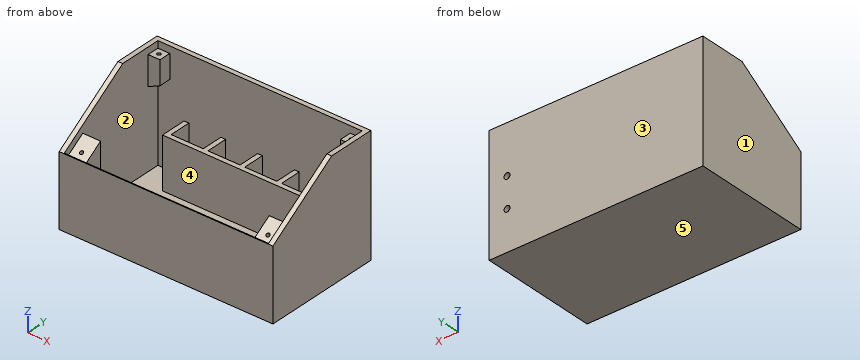
from build123d import *

# Parameters (mm, degrees)
ESBO_O1_W                = 180
ESBO_O1_H                = 100
ESBO_O1_W_2              = 172
ESBO_O1_H_2              = 92
RESSALTO_EXTRUS_O1_DEPTH = 100
ESBO_O2_W                = 180
ESBO_O2_H                = 100
RESSALTO_EXTRUS_O2_DEPTH = 4
RESSALTO_EXTRUS_O3_DEPTH = 43
CORTE_EXTRUS_O1_DEPTH    = 263
CHANFRO1_SIZE            = 6
CHANFRO1_SIZE2           = 4.326661531
ESBO_O5_W                = 10
ESBO_O5_H                = 20
RESSALTO_EXTRUS_O4_DEPTH = 10
ESBO_O6_R                = 1.5
CORTE_EXTRUS_O2_DEPTH    = 32
ESBO_O7_R                = 2.5
CORTE_EXTRUS_O3_DEPTH    = 32
CHANFRO3_SIZE            = 4.663076582
CHANFRO3_SIZE_2          = 10
CHANFRO4_SIZE            = 10
CHANFRO4_SIZE_2          = 4.663076582
RESSALTO_EXTRUS_O5_DEPTH = 15
RESSALTO_EXTRUS_O6_DEPTH = 15
CHANFRO5_SIZE2           = 15
CHANFRO5_SIZE            = 6.994614872
CHANFRO6_SIZE2           = 15
CHANFRO6_SIZE            = 6.994614872
ESBO_O10_R               = 1.5
CORTE_EXTRUS_O4_DEPTH    = 5
ESBO_O11_W               = 11
ESBO_O11_H               = 26
ESBO_O11_R               = 2
RESSALTO_EXTRUS_O7_DEPTH = 5


# Some blends are built 0.0001 mm under size
with BuildPart() as part:
    # Esboço1 → Ressalto-extrusão1 (new body)
    with BuildSketch(Plane.XY):
        with Locations((90, 50)):
            Rectangle(ESBO_O1_W, ESBO_O1_H)
        with Locations((90, 50)):
            Rectangle(ESBO_O1_W_2, ESBO_O1_H_2, mode=Mode.SUBTRACT)
    extrude(amount=RESSALTO_EXTRUS_O1_DEPTH)

    # Esboço2 → Ressalto-extrusão2 (add)
    with BuildSketch(Plane(origin=(0, 0, 0), x_dir=(-1, 0, 0), z_dir=(0, 0, -1))):
        with Locations((-90, 50)):
            Rectangle(ESBO_O2_W, ESBO_O2_H)
    extrude(amount=-RESSALTO_EXTRUS_O2_DEPTH)

    # Esboço3 → Ressalto-extrusão3 (add)
    with BuildSketch(Plane.XY.offset(4)):
        Polygon((30, 96), (30, 78), (57, 78), (57, 96), (61, 96), (61, 78), (88, 78), (88, 96), (92, 96), (92, 78), (119, 78), (119, 96), (123, 96), (123, 78), (150, 78), (150, 96), (154, 96), (154, 74), (26, 74), (26, 96), align=None)
    extrude(amount=RESSALTO_EXTRUS_O3_DEPTH)

    # Esboço4 → Corte-extrusão1 (cut)
    with BuildSketch(Plane.ZY):
        Polygon((60, 0), (100, 60), (100, 0), align=None)
    extrude(amount=-CORTE_EXTRUS_O1_DEPTH, mode=Mode.SUBTRACT)

    # Chanfro1
    chanfro1_edges = [part.edges().sort_by_distance(p)[0] for p in [
        (90, 4, 62.666666667),
    ]]
    chanfro1_side = [part.faces().sort_by_distance(p)[0] for p in [
        (90, 4, 33.333333333),
    ]]
    chamfer(chanfro1_edges, length=CHANFRO1_SIZE, length2=CHANFRO1_SIZE2, reference=chanfro1_side[0])

    # Esboço5 → Ressalto-extrusão4 (add)
    with BuildSketch(Plane.XZ.offset(-96)):
        with Locations((9, 84.2)):
            Rectangle(ESBO_O5_W, ESBO_O5_H)
        with Locations((171, 84.2)):
            Rectangle(ESBO_O5_W, ESBO_O5_H)
    extrude(amount=RESSALTO_EXTRUS_O4_DEPTH)

    # Esboço6 → Corte-extrusão2 (cut)
    with BuildSketch(Plane.XY.offset(94.2)):
        with Locations((171, 91)):
            Circle(ESBO_O6_R)
        with Locations((9, 91)):
            Circle(ESBO_O6_R)
    extrude(amount=-CORTE_EXTRUS_O2_DEPTH, mode=Mode.SUBTRACT)

    # Esboço7 → Corte-extrusão3 (cut)
    with BuildSketch(Plane.XZ.offset(-96)):
        with Locations(Location((165, 58.88, 0), (0, 0, 270))):
            Circle(ESBO_O7_R)
        with Locations(Location((165, 33.58, 0), (0, 0, 270))):
            Circle(ESBO_O7_R)
    extrude(amount=-CORTE_EXTRUS_O3_DEPTH, mode=Mode.SUBTRACT)

    # Chanfro3
    # the kernel refuses this chamfer: 10, 4.663076582 mm, written as the material it adds along each edge
    with BuildSketch(Plane(origin=(176, 96, 74.2), x_dir=(0.07481330637059742, 0, -0.9971975577536776), z_dir=(0, -1, 0))) as chanfro3_piece_1_section:
        Polygon((CHANFRO3_SIZE * 0.997197557657, -CHANFRO3_SIZE * 0.0748133063634), (-CHANFRO3_SIZE_2 * 0.0748133063706, -CHANFRO3_SIZE_2 * 0.997197557754), (0, 0), align=None)
    chanfro3_piece_1 = extrude(amount=10, mode=Mode.PRIVATE)
    chanfro3_piece_1 = split(chanfro3_piece_1, bisect_by=Plane(origin=(166, 91.000000816, 72.695597538), z_dir=(1, 0, 0)), keep=Keep.TOP, mode=Mode.PRIVATE)
    chanfro3_piece_1 = chanfro3_piece_1 - Plane(origin=(171, 91, 72.695597538), x_dir=(1, 0, 0), z_dir=(0, 0, 1)) * Cylinder(1.5, 60, mode=Mode.PRIVATE)
    add(chanfro3_piece_1)

    # Chanfro4
    # the kernel refuses this chamfer: 10, 4.663076582 mm, written as the material it adds along each edge
    with BuildSketch(Plane(origin=(4, 96, 74.2), x_dir=(0.9998669641130704, 0, 0.01631116413111014), z_dir=(0, -1, 0))) as chanfro4_piece_1_section:
        Polygon((CHANFRO4_SIZE * 0.999866964113, -CHANFRO4_SIZE * 0.0163111641311), (-CHANFRO4_SIZE_2 * 0.0163111641295, -CHANFRO4_SIZE_2 * 0.999866964017), (0, 0), align=None)
    chanfro4_piece_1 = extrude(amount=10, mode=Mode.PRIVATE)
    chanfro4_piece_1 = chanfro4_piece_1 - Plane(origin=(9, 91, 72.695597727), x_dir=(1, 0, 0), z_dir=(0, 0, 1)) * Cylinder(1.5, 60, mode=Mode.PRIVATE)
    chanfro4_piece_1 = split(chanfro4_piece_1, bisect_by=Plane(origin=(14, 91.000000829, 72.695597727), z_dir=(-1, 0, 0)), keep=Keep.TOP, mode=Mode.PRIVATE)
    add(chanfro4_piece_1)

    # Esboço8 → Ressalto-extrusão5 (add)
    with BuildSketch(Plane.ZY.offset(-176)):
        Polygon((56.224748388, 4), (66.358081721, 19.2), (43.224748388, 19.2), (43.224748388, 4), align=None)
    extrude(amount=RESSALTO_EXTRUS_O5_DEPTH)

    # Esboço9 → Ressalto-extrusão6 (add)
    with BuildSketch(Plane(origin=(4, 0, 0), x_dir=(0, 0, -1), z_dir=(1, 0, 0))):
        Polygon((-43.224748388, 19.2), (-66.358081721, 19.2), (-56.224748388, 4), (-43.224748388, 4), align=None)
    extrude(amount=RESSALTO_EXTRUS_O6_DEPTH)

    # Chanfro5
    chanfro5_edges = [part.edges().sort_by_distance(p)[0] for p in [
        (176, 11.6, 43.224748388),
    ]]
    chanfro5_side = [part.faces().sort_by_distance(p)[0] for p in [
        (176, 11.6, 43.08485609),
    ]]
    chamfer(chanfro5_edges, length=CHANFRO5_SIZE - 0.0001, length2=CHANFRO5_SIZE2 - 0.0001, reference=chanfro5_side[0])  # a hair under: the kernel refuses the full size

    # Chanfro6
    chanfro6_edges = [part.edges().sort_by_distance(p)[0] for p in [
        (4, 11.6, 43.224748388),
    ]]
    chanfro6_side = [part.faces().sort_by_distance(p)[0] for p in [
        (4, 11.6, 43.08485609),
    ]]
    chamfer(chanfro6_edges, length=CHANFRO6_SIZE - 0.0001, length2=CHANFRO6_SIZE2 - 0.0001, reference=chanfro6_side[0])  # a hair under: the kernel refuses the full size

    # Esboço10 → Corte-extrusão4 (cut)
    with BuildSketch(Plane(origin=(0, -24.719114641, 37.078671961), x_dir=(1, 0, 0), z_dir=(0, -0.5547001962252299, 0.8320502943378433))):
        with Locations(Location((11.5, 40.361212297, 0), (0, 0, 270))):
            Circle(ESBO_O10_R)
        with Locations(Location((168.5, 40.375568889, 0), (0, 0, 270))):
            Circle(ESBO_O10_R)
    extrude(amount=-CORTE_EXTRUS_O4_DEPTH, mode=Mode.SUBTRACT)

    # Esboço11 → Ressalto-extrusão7 (add)
    # profile 1 of 2: a face of its own
    with BuildSketch(Plane.XY.offset(4)):
        with Locations((122.5, 39)):
            Rectangle(ESBO_O11_W, ESBO_O11_H)
        with Locations((122.5, 45.5)):
            Circle(ESBO_O11_R, mode=Mode.SUBTRACT)
        with Locations((122.5, 32.5)):
            Circle(ESBO_O11_R, mode=Mode.SUBTRACT)
    # profile 2 of 2: a face of its own
    with BuildSketch(Plane.XY.offset(4)):
        with Locations((86.5, 39)):
            Rectangle(ESBO_O11_W, ESBO_O11_H)
        with Locations((86.5, 45.5)):
            Circle(ESBO_O11_R, mode=Mode.SUBTRACT)
        with Locations((86.5, 32.5)):
            Circle(ESBO_O11_R, mode=Mode.SUBTRACT)
    extrude(amount=RESSALTO_EXTRUS_O7_DEPTH)


solid = part.part
The listing builds one solid part. Answer for the finished solid, in the listing's coordinates (mm). Face numbers are marked on the shaded views. A direction names the side the tool comes from. Coordinates: 2 decimals unless noted, no trailing zeros. Write each loop counter-clockwise with the first axis right and the second up, starting at its lowest first coordinate (ties: lowest second). Pieces come first, ordered by that corner, then holes. Notation, with made-up numbers: (1.5, 59.5) - (47.5, 59.5) arc R25 cw to (47.5, 80.5) - close; hole circle Ø3 at (-4, 62). An arc over 180 degrees is marked (long way). Return JSON: item names as keys, results as strings.
1. For a pull along Y with two mould halves and no side action, classify the marked faces 1, 2 and 3 as +Y half, -Y half, draft (parallel to the pull), parting line (faces both ways), or undercut.
Final values:
{"face 1": "draft", "face 2": "undercut", "face 3": "+Y half"}
2. The part is cut by section A-A on z = 33.58. Count the separate pieces of the cut face and the enclosed holes in it, then the cut area to 3 significant figures.
Final values:
{"separate pieces": "1", "enclosed holes": "4", "area": "3,030 mm^2"}
3. Each of these flat-tipped pins is pushed along its axis until it touches: pin 1 Ø3.5 at (x, y) = (9, 91) entering from +Z; pin 2 Ø3 at (x, z) = (52.5, 73.5) entering from -Y; pin 3 Ø11 at (x, y) = (89.5, 81) entering from +Z. Where does it stop, or does it pass through?
Final values:
{"pin 1": "z = 94.2", "pin 2": "y = 96", "pin 3": "z = 47"}
4. The part is cut by section C-C on x = 21.5. Determine the outline of the cut face in (y, z).
Final values:
{"outline": "(0, 0) - (100, 0) - (100, 100) - (96, 100) - (96, 4) - (4, 4) - (4, 56.67) - (0.4, 60.27) - (0, 60) - close"}
5. The part is cut by section B-B on z = 16. Determine the outline of the cut face in (x, y), then the cut area to 3 significant figures.
Final values:
{"outline": "(0, 0) - (180, 0) - (180, 100) - (0, 100) - close; hole (4, 4) - (176, 4) - (176, 96) - (154, 96) - (154, 74) - (26, 74) - (26, 96) - (4, 96) - close; hole (30, 78) - (57, 78) - (57, 96) - (30, 96) - close; hole (61, 78) - (88, 78) - (88, 96) - (61, 96) - close; hole (92, 78) - (119, 78) - (119, 96) - (92, 96) - close; hole (123, 78) - (150, 78) - (150, 96) - (123, 96) - close", "area": "3,050 mm^2"}
6. Which of the six approach directions +Z, -Z, +X, -X, +Y, -Y give full straight-line access (tool end or side, diameter ignored) to the marked faces 4 and 5?
Final values:
{"face 4": "+Z", "face 5": "-Z, +X, -X, +Y, -Y"}
7. The part is cut by section D-D on y = 64.5. Determine the outline of the cut face in (x, z), then the cut area to 3 significant figures.
Final values:
{"outline": "(0, 0) - (180, 0) - (180, 100) - (176, 100) - (176, 4) - (4, 4) - (4, 100) - (0, 100) - close", "area": "1,490 mm^2"}
8. Consider line 1 along Z through (x, y) = (165, 98.6); line 2 along Y through (x, z) = (93, 41.5); line 3 along X through (y, z) = (75.5, 35.5). Determine where each line is inside the solid, lowest interval first.
Final values:
{"line 1": "0 to 31.08, 36.08 to 56.38, 61.38 to 100", "line 2": "0 to 4, 74 to 78, 96 to 100", "line 3": "0 to 4, 26 to 154, 176 to 180"}
